Design review of the part built by this model. Coordinates are the model's own, in mm. Give positions to 0.01 mm unless a question says otherwise; leave off trailing zeros. Loops run counter-clockwise (first coordinate to the right, second up) from the corner with the lowest first, then second, coordinate; pieces in that order, holes last. Notation, with made-up numbers: (-39.75, -4.75) -> (-7.75, -4.75) arc R15 cw to (-7.75, 9.25) -> close; hole circle Ø5 at (7.25, 87). An arc over 180 degrees is marked (long way). Answer as CSV lines item,"result".
from build123d import *

# Parameters (mm, degrees)
SKETCH1_W               = 25.4
SKETCH1_H               = 50.8
SKETCH1_W_2             = 22.225
SKETCH1_H_2             = 47.625
BOSS_EXTRUDE1_DEPTH     = 635
CUT_EXTRUDE1_DEPTH      = 638.534940219
CUT_EXTRUDE1_DEPTH_BACK = 638.534940219
SKETCH2_R               = 14.3129


with BuildPart() as part:
    # Sketch1 → Boss-Extrude1 (new body)
    with BuildSketch(Plane.XY):
        with Locations((12.7, 25.4)):
            Rectangle(SKETCH1_W, SKETCH1_H)
        with Locations((12.7, 25.4)):
            Rectangle(SKETCH1_W_2, SKETCH1_H_2, mode=Mode.SUBTRACT)
    extrude(amount=BOSS_EXTRUDE1_DEPTH)

    # Sketch2 → Cut-Extrude1 (cut, two sides: drawn at the far end of the back side and taken through both)
    with BuildSketch(Plane(origin=(25.4, 0, 0), x_dir=(0, 0, -1), z_dir=(1, 0, 0)).offset(-CUT_EXTRUDE1_DEPTH_BACK)):
        with Locations((-25.4, 25.4)):
            Circle(SKETCH2_R)
        with Locations((-609.6, 25.4)):
            Circle(SKETCH2_R)
    extrude(amount=CUT_EXTRUDE1_DEPTH + CUT_EXTRUDE1_DEPTH_BACK, mode=Mode.SUBTRACT)


solid = part.part
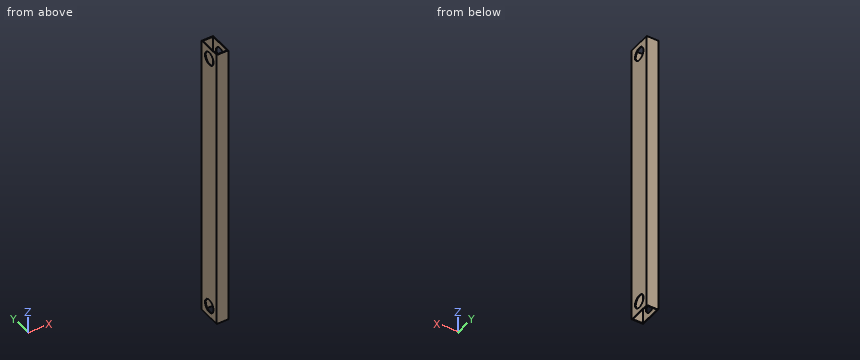
Q1. We need section B-B, the plane z = 323. State the section outline as (x, y) points, and give its area (3 significant figures).
Filled sheet:
outline,"(0, 0) -> (25.4, 0) -> (25.4, 50.8) -> (0, 50.8) -> close; hole (1.59, 1.59) -> (23.81, 1.59) -> (23.81, 49.21) -> (1.59, 49.21) -> close"
area,"232 mm^2"
Q2. We need section D-D, the plane y = 25.4. State the section outline as (x, z) points.
Filled sheet:
outline,"(0, 0) -> (1.59, 0) -> (1.59, 11.09) -> (0, 11.09) -> close; (0, 39.71) -> (1.59, 39.71) -> (1.59, 595.29) -> (0, 595.29) -> close; (0, 623.91) -> (1.59, 623.91) -> (1.59, 635) -> (0, 635) -> close; (23.81, 0) -> (25.4, 0) -> (25.4, 11.09) -> (23.81, 11.09) -> close; (23.81, 39.71) -> (25.4, 39.71) -> (25.4, 595.29) -> (23.81, 595.29) -> close; (23.81, 623.91) -> (25.4, 623.91) -> (25.4, 635) -> (23.81, 635) -> close"
Q3. To check wall thickness, follow probe 1 along Z at (x, y) = (0.8, 25.4); probe 2 along X at (y, z) = (9.5, 54.5); probe 3 along Y at (x, z) = (14.75, 42). State the ranges of each line that lie inside material, in increasing order. Write a range as from..to.
Filled sheet:
probe 1,"z = 0..11.09, 39.71..595.29, 623.91..635"
probe 2,"x = 0..1.59, 23.81..25.4"
probe 3,"y = 0..1.59, 49.21..50.8"
Q4. We need section C-C, the plane x = 18.25. State the section outline as (y, z) points, and give its area (3 significant figures).
Filled sheet:
outline,"(0, 0) -> (1.59, 0) -> (1.59, 635) -> (0, 635) -> close; (49.21, 0) -> (50.8, 0) -> (50.8, 635) -> (49.21, 635) -> close"
area,"2,020 mm^2"
Q5. We need section A-A, the plane z = 25.4. State the section outline as (x, y) points, and give its area (3 significant figures).
Filled sheet:
outline,"(0, 0) -> (25.4, 0) -> (25.4, 11.09) -> (23.81, 11.09) -> (23.81, 1.59) -> (1.59, 1.59) -> (1.59, 11.09) -> (0, 11.09) -> close; (0, 39.71) -> (1.59, 39.71) -> (1.59, 49.21) -> (23.81, 49.21) -> (23.81, 39.71) -> (25.4, 39.71) -> (25.4, 50.8) -> (0, 50.8) -> close"
area,"141 mm^2"
